Read the model definition and answer for the solid it produces. Units are mm, in the model's axes. Face numbers are marked on the shaded views. A direction names the side the tool comes from. Coordinates: 2 decimals unless noted, no trailing zeros. Loops run counter-clockwise (first coordinate to the right, second up) from the corner with the lowest first, then second, coordinate; pieces in that order, holes last.
Q1. The mould has two halves that part along Y. Classify the marked faces 1, 2, 3 and 4: pulls with the +Y half, pulls with the -Y half, needs draft (parallel to the pull), parting line crosses it, or undercut.
Q2. Section A-A (x = -27) is taken. Give the vertices of the cut face in (y, z).
Q3. Section D-D (x = 10) is taken. Give the vertices of the cut face in (y, z).
Q4. Straight lines are drawn through the part: line 1 (Y direction, x = 21.5, z = 7.5); line 2 (X direction, y = 0, z = 10.25); line 3 (X direction, y = -19, z = 1). For each, find the intervals that lie inside material, in ascending order.
Q5. Which of the six approach directions +Z, -Z, +X, -X, +Y, -Y give full straight-line access (tool end or side, diameter ignored) to the marked faces 5, 6 and 7?
Q6. Flat-ended cylindrical pins translate along their axes: P1, Ø4, axis at y = -20, z = 5.5, coming from the -X side; P2, Ø6, axis at y = 0, z = 7, coming from the +X side; P3, Ø3, axis at y = 9.5, z = 8, coming from the +X side. Find the tip coordinate at first contact, or state that the pin passes through.
Q7. Section B-B (y = 0) is taken. Give the vertices of the cut face in (x, z), then the cut area to 3 significant figures.
Q8. Section C-C (z = 5.25) is taken. Give the vertices of the cut face in (x, y), then the cut area to 3 significant figures.
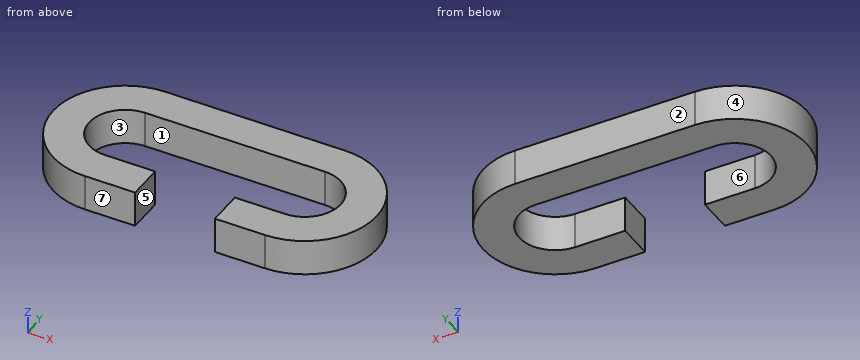
from build123d import *

# Parameters (mm, degrees)
F1_DEPTH = 12.7


# Not quite as in the source:
# - a feature of the source that left no trace in its solid (it failed there, or was rolled back) is left out


with BuildPart() as f1:
    # F0 (on Top) → F1 (new body)
    with BuildSketch(Plane.XY):
        with BuildLine():
            ThreePointArc((31.75, 12.7), (44.45, 0), (31.75, -12.7))
            Line((31.75, -12.7), (14.0969706699, -12.7))
            Line((14.0969706699, -12.7), (14.0969706699, -25.4))
            Line((14.0969706699, -25.4), (31.75, -25.4))
            ThreePointArc((31.75, -25.4), (57.15, 0), (31.75, 25.4))
            Line((31.75, 25.4), (0, 25.4))
            Line((0, 25.4), (-31.75, 25.4))
            ThreePointArc((-31.75, 25.4), (-57.15, 0), (-31.75, -25.4))
            Line((-31.75, -25.4), (-14.0969706699, -25.4))
            Line((-14.0969706699, -25.4), (-14.0969706699, -12.7))
            Line((-14.0969706699, -12.7), (-31.75, -12.7))
            ThreePointArc((-31.75, -12.7), (-44.45, 0), (-31.75, 12.7))
            Line((-31.75, 12.7), (0, 12.7))
            Line((0, 12.7), (31.75, 12.7))
        make_face()
    extrude(amount=F1_DEPTH)


solid = f1.part
Numbers:
1. face 1: undercut
1. face 2: pulls with the +Y half
1. face 3: undercut
1. face 4: parting line crosses it
2. outline: (-25.4, 0) - (-12.7, 0) - (-12.7, 12.7) - (-25.4, 12.7) - close; (12.7, 0) - (25.4, 0) - (25.4, 12.7) - (12.7, 12.7) - close
3. outline: (12.7, 0) - (25.4, 0) - (25.4, 12.7) - (12.7, 12.7) - close
4. line 1: y = -25.4 to -12.7, 12.7 to 25.4
4. line 2: x = -57.15 to -44.45, 44.45 to 57.15
4. line 3: x = -48.61 to -14.1, 14.1 to 48.61
5. face 5: +Z, -Z, -Y
5. face 6: +Z, -Z
5. face 7: +Z, -Z, +X, -X, -Y
6. P1: stops at x = -49.67
6. P2: stops at x = 57.15
6. P3: stops at x = 55.86
7. outline: (-57.15, 0) - (-44.45, 0) - (-44.45, 12.7) - (-57.15, 12.7) - close; (44.45, 0) - (57.15, 0) - (57.15, 12.7) - (44.45, 12.7) - close
7. area: 323 mm2
8. outline: (-31.75, -25.4) - (-14.1, -25.4) - (-14.1, -12.7) - (-31.75, -12.7) arc R12.7 cw to (-31.75, 12.7) - (31.75, 12.7) arc R12.7 cw to (31.75, -12.7) - (14.1, -12.7) - (14.1, -25.4) - (31.75, -25.4) arc R25.4 ccw to (31.75, 25.4) - (-31.75, 25.4) arc R25.4 ccw to start
8. area: 2,770 mm2
